from build123d import *

# Parameters (mm, degrees)
SKETCH1_R           = 6.35
BOSS_EXTRUDE1_DEPTH = 6.35


with BuildPart() as part:
    # Sketch1 → Boss-Extrude1 (new body)
    with BuildSketch(Plane.XY):
        with BuildLine():
            Line((-8.248891971, 37.758067884), (-36.823891971, -11.735283942))
            ThreePointArc((-36.823891971, -11.735283942), (-36.823891971, -21.260283942), (-28.575, -26.022783942))
            Line((-28.575, -26.022783942), (28.575, -26.022783942))
            ThreePointArc((28.575, -26.022783942), (36.823891971, -21.260283942), (36.823891971, -11.735283942))
            Line((36.823891971, -11.735283942), (8.248891971, 37.758067884))
            ThreePointArc((8.248891971, 37.758067884), (0, 42.520567884), (-8.248891971, 37.758067884))
        make_face()
        Circle(SKETCH1_R, mode=Mode.SUBTRACT)
        with Locations((-28.575, -16.497783942)):
            Circle(SKETCH1_R, mode=Mode.SUBTRACT)
        with Locations((0, 32.995567884)):
            Circle(SKETCH1_R, mode=Mode.SUBTRACT)
        with Locations((28.575, -16.497783942)):
            Circle(SKETCH1_R, mode=Mode.SUBTRACT)
    extrude(amount=BOSS_EXTRUDE1_DEPTH)


solid = part.part
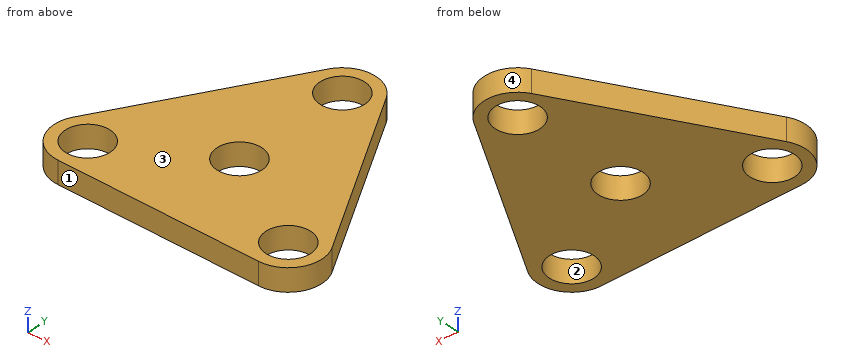
Can you work these out from the model? Positions are in its coordinate system, mm. Face numbers are marked on the shaded views. Coordinates: 2 decimals unless noted, no trailing zeros. Write each loop counter-clockwise with the first axis right and the second up, starting at its lowest first coordinate (ties: lowest second). Pieces come first, ordered by that corner, then holes.
Q1. Imagine slicing it at C-C, the plane y = 0. List the corners of the cut face in (x, z) for me.
Results found:
outline: (-30.05, 0) - (-6.35, 0) - (-6.35, 6.35) - (-30.05, 6.35) - close; (6.35, 0) - (30.05, 0) - (30.05, 6.35) - (6.35, 6.35) - close
Q2. Imagine slicing it at D-D, the plane z = 1.75. List the corners of the cut face in (x, y) for me (3 decimals).
Results found:
outline: (-36.824, -11.735) arc R9.525 ccw to (-28.575, -26.023) - (28.575, -26.023) arc R9.525 ccw to (36.824, -11.735) - (8.249, 37.758) arc R9.525 ccw to (-8.249, 37.758) - close; hole circle Ø12.7 at (-28.575, -16.498); hole circle Ø12.7 at (0, 0); hole circle Ø12.7 at (0, 32.996); hole circle Ø12.7 at (28.575, -16.498)
Q3. Imagine slicing it at A-A, the plane x = 0. List the corners of the cut face in (y, z) for me.
Results found:
outline: (-26.02, 0) - (-6.35, 0) - (-6.35, 6.35) - (-26.02, 6.35) - close; (6.35, 0) - (26.65, 0) - (26.65, 6.35) - (6.35, 6.35) - close; (39.35, 0) - (42.52, 0) - (42.52, 6.35) - (39.35, 6.35) - close
Q4. Imagine slicing it at B-B, the plane x = 32. List the corners of the cut face in (y, z) for me.
Results found:
outline: (-25.39, 0) - (-21.84, 0) - (-21.84, 6.35) - (-25.39, 6.35) - close; (-11.15, 0) - (-3.38, 0) - (-3.38, 6.35) - (-11.15, 6.35) - close
Q5. Please list where these lines run through material, in increasing order: L1, parallel to X at y = -14, z = 1.25; L2, parallel to X at y = -19.5, z = 2.5; L3, parallel to Y at x = 3, z = 4.
Results found:
L1: x = -37.77 to -34.41, -22.74 to 22.74, 34.41 to 37.77
L2: x = -37.61 to -34.17, -22.98 to 22.98, 34.17 to 37.61
L3: y = -26.02 to -5.6, 5.6 to 27.4, 38.59 to 42.04
Q6. For P1, Ø2, axis at y = -8, z = 4, coming from the -X side, with a flat end and sliding along its axis, tell me the tip position at first contact or that it passes through.
Results found:
P1: stops at x = -35.24
Q7. If we mould it in two halves opening along Y, with no side actions, what happens to the marked faces 1, 2, 3 and 4? For each: +Y half, -Y half, draft (parallel to the pull), parting line (faces both ways), or undercut.
Results found:
face 1: -Y half
face 2: undercut
face 3: draft
face 4: +Y half
